```python
from build123d import *

# Parameters (mm, degrees)
F0_W     = 63.5
F0_H     = 63.5
F1_DEPTH = 31.75
F2_T     = -2.54
F3_DEPTH = 2.541
F4_W     = 58.42
F4_H     = 58.42
F5_DEPTH = 63.501
F6_W     = 58.42
F6_H     = 58.42
F7_DEPTH = 63.501


with BuildPart() as f1:
    # F0 (on Top) → F1 (new body, symmetric)
    with BuildSketch(Plane.XY):
        Rectangle(F0_W, F0_H)
    extrude(amount=F1_DEPTH, both=True)

    # F2
    f2_openings = [f1.faces().sort_by_distance(p)[0] for p in [
        (-31.75, 0, 0),
    ]]
    offset(amount=F2_T, openings=f2_openings)

    # F3 (cut, through all): a face of the model
    f3_faces = [f1.faces().sort_by_distance(p)[0] for p in [
        (29.21, 0, 0),
    ]]
    extrude(f3_faces, amount=-F3_DEPTH, mode=Mode.SUBTRACT)

    # F4 (on face) → F5 (cut, through all)
    with BuildSketch(Plane.XY.offset(31.75)):
        Rectangle(F4_W, F4_H)
    extrude(amount=-F5_DEPTH, mode=Mode.SUBTRACT)

    # F6 (on face) → F7 (cut, through all)
    with BuildSketch(Plane(origin=(0, 31.75, 0), x_dir=(-1, 0, 0), z_dir=(0, 1, 0))):
        Rectangle(F6_W, F6_H)
    extrude(amount=-F7_DEPTH, mode=Mode.SUBTRACT)


solid = f1.part
```
Geometry: final body of the model. Coordinates: model frame, mm. A direction names the side the tool comes from. Coordinates: 2 decimals unless noted, no trailing zeros. Order: outer loops, then holes, each group sorted by start corner. A loop starts at its lowest first (then second) coordinate and runs counter-clockwise, first axis right, second up. Notation, with made-up numbers: (-27.5, -12) - (-20.5, -12) arc R10 cw to (-20.5, 7) - close; hole circle Ø10 at (57, 29). An arc over 180 degrees is marked (long way). Write each question's results on one line, items separated by ' | '.
(1) Mould query, pull axis X, two halves, no side actions, for faces 5 (the face through (0, 29.21, -30)), 6 (the face through (-3, 31.75, -30)), 7 (the face through (31.75, -3, -30)). Classes: +X half, -X half, draft (parallel to the pull), parting line (faces both ways), or undercut.
Values found:
face 5: undercut | face 6: draft | face 7: +X half
(2) Section query A-A, the plane z = 16. Return the cut outline in (x, y).
Values found:
outline: (-31.75, -31.75) - (-29.21, -31.75) - (-29.21, -29.21) - (-31.75, -29.21) - close; (-31.75, 29.21) - (-29.21, 29.21) - (-29.21, 31.75) - (-31.75, 31.75) - close; (29.21, -31.75) - (31.75, -31.75) - (31.75, -29.21) - (29.21, -29.21) - close; (29.21, 29.21) - (31.75, 29.21) - (31.75, 31.75) - (29.21, 31.75) - close
(3) First-contact query: pin 1 Ø10 at (x, y) = (-1.5, -19.5) entering from +Z. Flat tip, straight axial feed; report the tip coordinate or a pass-through.
Values found:
pin 1: passes through
(4) Set-up query: faces 1 (the face through (-29.21, -30, 0)), 2 (the face through (0, -29.21, -30)), 3 (the face through (-3, -31.75, -30)), 4 (the face through (-30, 29.21, 0)). Return all of +Z, -Z, +X, -X, +Y, -Y with unobstructed straight access to the full face (end or side cutting, diameter ignored); none if empty.
Values found:
face 1: +Y, -Y | face 2: +Z, -Z | face 3: +Z, -Z, +X, -X, -Y | face 4: +X, -X
